Geometry check sheet. Reference: the model listing, model coordinates, mm. Face numbers are marked on the shaded views. Coordinates: 2 decimals unless noted, no trailing zeros. Write each loop counter-clockwise with the first axis right and the second up, starting at its lowest first coordinate (ties: lowest second). Pieces come first, ordered by that corner, then holes. Notation, with made-up numbers: M 28.5,17.5 L 43.5,17.5 A18 cw 43.5,38.5 Z; hole C -10.5,80 d7. An arc over 180 degrees is marked long. Put each result on its own line as item: value. Start each with the question number.
1) Scan lines: line 1 along X through (y, z) = (-80, -0.25); line 2 along X through (y, z) = (-62, -2.15); line 3 along Z through (x, y) = (-0.25, -36). Record each from-to range of solid material in increasing order.
2) Gauge pin test, flat end, axial feed: pin 1 (1 mm diameter, centred on y = -27.5, z = -1, fed in from -X). Record the tip position at first contact, or that the pin passes through.
3) Cross-section at B-B on x = 0. Record the cut outline in (y, z).
4) Mould release check, pull along X, two halves, no side actions. Record for the marked faces 1 and 2: released by +X, released by -X, zero draft, split by the parting line, or undercut.
5) Cross-section at A-A on y = -35. Record the cut outline in (x, z), plus the area to 3 significant figures.
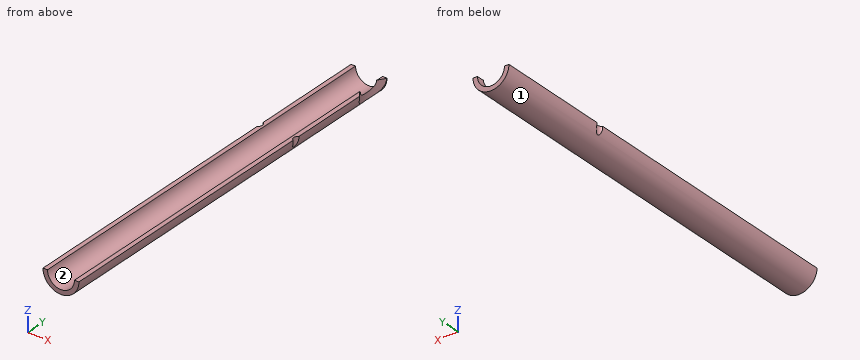
from build123d import *

# Parameters (mm, degrees)
F0_R          = 4
F0_R_2        = 3
F1_DEPTH      = 89.8
F3_DEPTH      = 96.4
F4_R          = 6
F5_DEPTH      = 25
F5_DEPTH_BACK = 25
F6_R          = 1
F7_DEPTH      = 25
F7_DEPTH_BACK = 25


with BuildPart() as f1:
    # F0 (on Front) → F1 (new body)
    with BuildSketch(Plane.XZ):
        Circle(F0_R)
        Circle(F0_R_2, mode=Mode.SUBTRACT)
    extrude(amount=F1_DEPTH)

    # F2 (on face) → F3 (cut)
    with BuildSketch(Plane.XZ.offset(89.8)):
        Polygon((-5.919513, 0), (0, 0), (6.079678, 0), (6.079678, 7.445201), (-5.919513, 7.445201), align=None)
    extrude(amount=-F3_DEPTH, mode=Mode.SUBTRACT)

    # F4 (on Top) → F5 (cut, two sides)
    with BuildSketch(Plane.XY) as f5_sk:
        with Locations((8.5, -4.1)):
            Circle(F4_R)
    extrude(amount=-F5_DEPTH, mode=Mode.SUBTRACT)
    extrude(f5_sk.sketch, amount=-F5_DEPTH_BACK, mode=Mode.SUBTRACT)

    # F6 (on face) → F7 (cut, two sides)
    with BuildSketch(Plane.XY) as f7_sk:
        with Locations((4.5, -26.5)):
            Circle(F6_R)
        with Locations((-4.5, -26.5)):
            Circle(F6_R)
    extrude(amount=-F7_DEPTH, mode=Mode.SUBTRACT)
    extrude(f7_sk.sketch, amount=-F7_DEPTH_BACK, mode=Mode.SUBTRACT)


solid = f1.part
Answer key:
1. line 1: x = -3.99 to -2.99, 2.99 to 3.99
1. line 2: x = -3.37 to -2.09, 2.09 to 3.37
1. line 3: z = -3.99 to -2.99
2. pin 1: stops at x = -3.97
3. outline: M -89.8,-4 L 0,-4 L 0,-3 L -89.8,-3 Z
4. face 1: split by the parting line
4. face 2: undercut
5. outline: M -4,0 A4 ccw 4,0 L 3,0 A3 cw -3,0 Z
5. area: 11.0 mm²
